Work out the finished part from the listing and answer in its coordinate system (mm). Coordinates: 2 decimals unless noted, no trailing zeros. Order: outer loops, then holes, each group sorted by start corner. A loop starts at its lowest first (then second) coordinate and runs counter-clockwise, first axis right, second up. Notation, with made-up numbers: (20, 80) -> (67, 80) arc R28 ccw to (67, 98) -> close; hole circle Ø5 at (-21, 23.25). An arc over 180 degrees is marked (long way). Answer as CSV lines item,"result". Start each with the question number.
Item 1: This flat-tipped pin is pushed along its axis until it touches: pin 1 Ø2 at (y, z) = (599, 2.5) entering from -X. Where does it stop, or does it pass through?
Item 2: Section A-A (y = 1335) is taken. Write down the section's boundary in (x, z), then the cut area to 3 significant figures.
Item 3: Straight lines are drawn through the part: L1, parallel to Y at x = -92.5, z = 0.2; L2, parallel to Y at x = -105, z = 2.4; L3, parallel to X at y = 602, z = 1.25. For each, find the intervals that lie inside material, in ascending order.
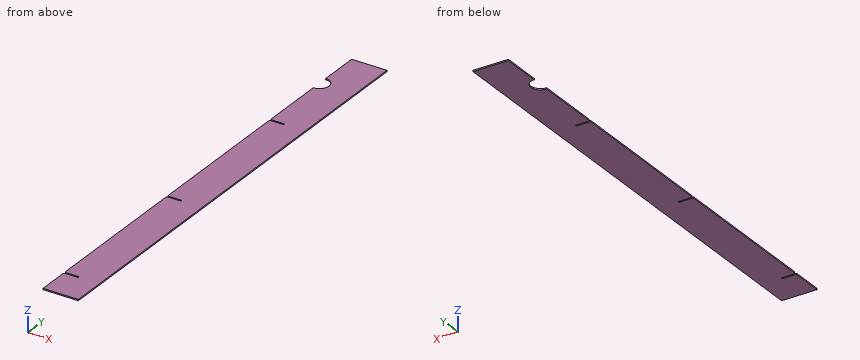
Autodesk Inventor part; units mm, degrees
ref_plane "YZ Plane" through (0, 0, 0) normal (1, 0, 0) x (0, 1, 0)
ref_plane "XZ Plane" through (0, 0, 0) normal (0, 1, 0) x (-1, 0, 0)
ref_plane "XY Plane" through (0, 0, 0) normal (0, 0, 1) x (1, 0, 0)
sketch "Sketch1" plane through (0, 0, 0) normal (0, 0, 1) x (1, 0, 0)
  line L0 (0, 1490) -> (-110.8614, 1490)
  line L1 (-110.8614, 1490) -> (-110.8614, 0)
  line L2 (-110.8614, 0) -> (0, 0)
  line L3 (0, 0) -> (0, 1490)
  line L4 (-110.8614, 100) -> (-66, 100)
  line L5 (-66, 100) -> (-66, 105)
  line L6 (-66, 105) -> (-110.8614, 105)
  line L7 (-110.8614, 105) -> (-110.8614, 100)
  line L8 (-110.8614, 596.6667) -> (-66, 596.6667)
  line L9 (-66, 596.6667) -> (-66, 601.6667)
  line L10 (-66, 601.6667) -> (-110.8614, 601.6667)
  line L11 (-110.8614, 601.6667) -> (-110.8614, 596.6667)
  line L12 (-110.8614, 1093.3333) -> (-66, 1093.3333)
  line L13 (-66, 1093.3333) -> (-66, 1098.3333)
  line L14 (-66, 1098.3333) -> (-110.8614, 1098.3333)
  line L15 (-110.8614, 1098.3333) -> (-110.8614, 1093.3333)
  circle A0 centre (-110.8614, 1335) radius 30
  point P0 (-110.8614, 1098.3333)
  point P1 (-110.8614, 1093.3333)
  point P2 (-110.8614, 601.6667)
  point P3 (-110.8614, 596.6667)
  point P4 (-110.8614, 105)
  point P5 (-110.8614, 1365)
  point P6 (-110.8614, 1305)
  dimension "d0" = 1490
  dimension "d1" = 110.8614
  dimension "d2" = 5
  dimension "d4" = 100
  dimension "d7" = 496.6667
  dimension "d23" = 66
  dimension "d29" = 60
  dimension "d30" = 1335
extrude "Plate1" add sketch "Sketch1" along normal blind 4 contours L3 L2 L1 L4 L5 L6 L8 L9 L10 L12 L13 L14 A0 L0
chamfer "Corner Chamfer1" distance 3 angle 45 6 edges at (-110.8614, 100, 2) (-110.8614, 105, 2) (-110.8614, 596.6667, 2) (-110.8614, 601.6667, 2) (-110.8614, 1098.3333, 2) (-110.8614, 1093.3333, 2)
equation "\"d0\" = Стрингер_длина"
equation "\"d1\" = стрингер_глубина_8"
equation "\"d2\" = паз_под_стрингер_толщина"
equation "\"d7\" = Шаг_шпангоутов"
equation "\"d23\" = паз_под_стрингер_глубина - Thickness"
equation "\"d29\" = 2 * радиус_выреза_под_сварку"
equation "\"d12\" = Thickness"
equation "\"BendRadius\" = Thickness"
equation "\"BendReliefWidth\" = Thickness"
equation "\"BendReliefDepth\" = 0.5 * Thickness"
equation "\"CornerReliefSize\" = 4 * Thickness"
equation "\"MinimumRemnant\" = 2 * Thickness"
equation "\"TransitionRadius\" = BendRadius"
equation "\"JacobiRadiusSize\" = BendRadius"
equation "\"GapSize\" = Thickness"
properties part number "01014 GBK stringer C8" material "Steel"
Checked values:
1,pin 1,"stops at x = -66"
2,outline,"(-80.86, 0) -> (0, 0) -> (0, 4) -> (-80.86, 4) -> close"
2,area,"323 mm^2"
3,L1,"y = 0 to 100, 105 to 596.67, 601.67 to 1093.33, 1098.33 to 1311.28, 1358.72 to 1490"
3,L2,"y = 0 to 100, 105 to 596.67, 601.67 to 1093.33, 1098.33 to 1305.58, 1364.42 to 1490"
3,L3,"x = -108.19 to 0"
